```python
from build123d import *

# Parameters (mm, degrees)
F0_R           = 1.5
F0_R_2         = 4.7625
F1_DEPTH       = 6.35
F2_D           = 2.5
F2_CSINK_D     = 4.7
F2_CSINK_ANGLE = 90
F4_D           = 2.05
F4_DEPTH       = 12.5
F4_TIP         = 0.6158821345
F5_D           = 2
F5_DEPTH       = 8
F5_TIP         = 0.600860619
F7_D           = 2
F7_DEPTH       = 8
F7_TIP         = 0.600860619


# Not quite as in the source:
# - a length typed as a fraction of an inch, garbled in the dataset ("3 / 203.2 mm" for 3/8 in), is restored


with BuildPart() as f1:
    # F0 (on Top) → F1 (new body)
    with BuildSketch(Plane.XY):
        with BuildLine():
            Line((28, 15), (-12.25, 15))
            ThreePointArc((-12.25, 15), (-26.35, 0), (-12.25, -15))
            Line((-12.25, -15), (28, -15))
            Line((28, -15), (28, -7.5))
            Line((28, -7.5), (21.65, -7.5))
            Line((21.65, -7.5), (21.65, 7.5))
            Line((21.65, 7.5), (28, 7.5))
            Line((28, 7.5), (28, 15))
        make_face()
        with Locations((0, -6)):
            Circle(F0_R, mode=Mode.SUBTRACT)
        with Locations((-18.5013860464, 0)):
            Circle(F0_R_2, mode=Mode.SUBTRACT)
        with BuildLine():
            ThreePointArc((-7.5, 0), (-6, 1.5), (-4.5, 0))
            ThreePointArc((-4.5, 0), (-6, -1.5), (-7.5, 0))
        make_face(mode=Mode.SUBTRACT)
        with BuildLine():
            ThreePointArc((2.5, 0), (0, -2.5), (-2.5, 0))
            ThreePointArc((-2.5, 0), (0, 2.5), (2.5, 0))
        make_face(mode=Mode.SUBTRACT)
        with Locations((0, 6)):
            Circle(F0_R, mode=Mode.SUBTRACT)
        with Locations((6, 0)):
            Circle(F0_R, mode=Mode.SUBTRACT)
    extrude(amount=F1_DEPTH)

    # F2 (through all)
    with Locations(Plane(origin=(0, 0, 0), x_dir=(1, 0, 0), z_dir=(0, 0, -1))):
        with Locations((24.825, -11.25), (24.825, 11.25)):
            CounterSinkHole(F2_D / 2, F2_CSINK_D / 2, counter_sink_angle=F2_CSINK_ANGLE)

    # F4
    with Locations(Plane.YZ.offset(21.65)):
        with Locations((0, 3.175)):
            Hole(F4_D / 2, depth=F4_DEPTH)
            with Locations((0, 0, -(F4_DEPTH + F4_TIP / 2))):  # 118° drill point
                Cone(0, F4_D / 2, F4_TIP, mode=Mode.SUBTRACT)

    # F5
    with Locations(Plane(origin=(0, 0, 0), x_dir=(1, 0, 0), z_dir=(0, 0, -1))):
        with Locations((-9.7427857926, 5.625), (-9.7427857926, -5.625)):
            Hole(F5_D / 2, depth=F5_DEPTH)
            with Locations((0, 0, -(F5_DEPTH + F5_TIP / 2))):  # 118° drill point
                Cone(0, F5_D / 2, F5_TIP, mode=Mode.SUBTRACT)

    # F7
    with Locations(Plane.XY.offset(6.35)):
        with Locations((11.4125, -11.25), (11.4125, 11.25)):
            Hole(F7_D / 2, depth=F7_DEPTH)
            with Locations((0, 0, -(F7_DEPTH + F7_TIP / 2))):  # 118° drill point
                Cone(0, F7_D / 2, F7_TIP, mode=Mode.SUBTRACT)


solid = f1.part
```
Here's how the part is built. I have some questions about the finished solid (model axes, mm). A direction names the side the tool comes from. Give positions to 0.01 mm unless a question says otherwise; leave off trailing zeros. Order: outer loops, then holes, each group sorted by start corner. A loop starts at its lowest first (then second) coordinate and runs counter-clockwise, first axis right, second up. Notation, with made-up numbers: M -5.75,70 L 46.25,70 A22 cw 46.25,81 Z; hole C 86.5,-31.75 d5. An arc over 180 degrees is marked long. Use a Markdown table: item, result. Add a question column.
1. I need wall thicknesses on probe 1 along Y at (x, z) = (0, 3); probe 2 along Y at (x, z) = (2, 1.25); probe 3 along X at (y, z) = (11.5, 2.75). Which ranges of each line are inside material? Lowest first, please. Write a range as from..to.
2. Suppose I cut it at C-C (y = -3). List the corners of the cut face in (x, z) for me, and give its area (3 significant figures).
3. Suppose I cut it at B-B (z = 4.75). Give the number of separate pieces and of enclosed holes in the cut face, and give its area (3 significant figures).
4. For pin 1 Ø1.8 at (x, y) = (-9.74, 5.62) entering from -Z; pin 2 Ø3 at (x, y) = (11.41, 11.25) entering from -Z; pin 3 Ø1.5 at (y, z) = (-5, 2) entering from +X; pin 4 Ø1.8 at (y, z) = (0, 3.175) entering from +X, each with a flat end and sliding along its axis, tell me the tip position at first contact or that it passes through.
5. On a 3-axis mill with a long thin cutter (end or side, diameter ignored), from which of +Z, -Z, +X, -X, +Y, -Y can I reach the whole of each face in a straight line? I mean faces 4 (the flat face through (21.65, 0, 5)), 5 (the flat face through (28, 11, 3)). Say none if no direction works.
6. If we mould it in two halves opening along X, with no side actions, what happens to faces 1 (the cylindrical face through (15.31, 0.13, 4.19)), 2 (the conical face through (8.64, -0.02, 3.35)), 3 (the cylindrical face through (-0.325, 4.536, 3.131))? For each: +X half, -X half, draft (parallel to the pull), parting line (faces both ways), or undercut.
7. Suppose I cut it at A-A (x = -6). List the corners of the cut face in (y, z) for me, and give its area (3 significant figures).
Results list:
| question | item | result |
|---|---|---|
| 1 | probe 1 | y = -15..-7.5, -4.5..-2.5, 2.5..4.5, 7.5..15 |
| 1 | probe 2 | y = -15..-1.5, 1.5..15 |
| 1 | probe 3 | x = -21..10.44, 12.38..23.6, 26.05..28 |
| 2 | outline | M -26.05,0 L -22.2,0 L -22.2,6.35 L -26.05,6.35 Z; M -14.8,0 L 21.65,0 L 21.65,6.35 L -14.8,6.35 Z |
| 2 | area | 256 mm² |
| 3 | separate pieces | 1 |
| 3 | enclosed holes | 12 |
| 3 | area | 1,300 mm² |
| 4 | pin 1 | passes through |
| 4 | pin 2 | stops at z = 0 |
| 4 | pin 3 | stops at x = 21.65 |
| 4 | pin 4 | stops at x = 9.07 |
| 5 | face 4 | +Z, -Z, +X |
| 5 | face 5 | +Z, -Z, +X, +Y, -Y |
| 6 | face 1 | draft |
| 6 | face 2 | +X half |
| 6 | face 3 | undercut |
| 7 | outline | M -15,0 L -1.5,0 L -1.5,6.35 L -15,6.35 Z; M 1.5,0 L 15,0 L 15,6.35 L 1.5,6.35 Z |
| 7 | area | 171 mm² |
